```python
from build123d import *

# Parameters (mm, degrees)
FILLET1_R   = 0.1
FILLET2_R   = 0.15
HEX_2_DEPTH = 1.3


with BuildPart() as part:
    # BodySke → Base-Revolve (revolve)
    with BuildSketch(Plane.XY, mode=Mode.PRIVATE) as base_revolve_sk:
        Polygon((0, 0), (0, 2.75), (3, 2.75), (3, 1.5), (18.7195, 1.5), (19, 1.2195), (19, 0), align=None)
    revolve(base_revolve_sk.sketch.rotate(Axis((-31.75, 0, 0), (1, 0, 0)), 90), axis=Axis((-31.75, 0, 0), (1, 0, 0)))  # turned: the seam where the file's is

    # Fillet1
    fillet1_edges = [part.edges().sort_by_distance(p)[0] for p in [
        (3, 0, -1.5),
    ]]
    fillet(fillet1_edges, radius=FILLET1_R)

    # Fillet2
    fillet2_edges = [part.edges().sort_by_distance(p)[0] for p in [
        (0, 0, -2.75),
    ]]
    fillet(fillet2_edges, radius=FILLET2_R)

    # Sketch2 → Hex-PreBroach (revolve, cut)
    with BuildSketch(Plane.XY, mode=Mode.PRIVATE) as hex_prebroach_sk:
        Polygon((0, 1.28), (1.3, 1.28), (2.039008345, 0), (0, 0), align=None)
    revolve(hex_prebroach_sk.sketch.rotate(Axis((0, 0, 0), (1, 0, 0)), 90), axis=Axis((0, 0, 0), (1, 0, 0)), mode=Mode.SUBTRACT)  # turned: the seam where the file's is

    # Sketch3 → Hex 2 (cut)
    with BuildSketch(Plane(origin=(0, 0, 0), x_dir=(0, 0.5, 0.866025404), z_dir=(-1, 0, 0))):
        Polygon((0.739008345, 1.28), (-0.739008345, 1.28), (-1.478016689, 0), (-0.739008345, -1.28), (0.739008345, -1.28), (1.478016689, 0), align=None)
    extrude(amount=-HEX_2_DEPTH, mode=Mode.SUBTRACT)


solid = part.part
```
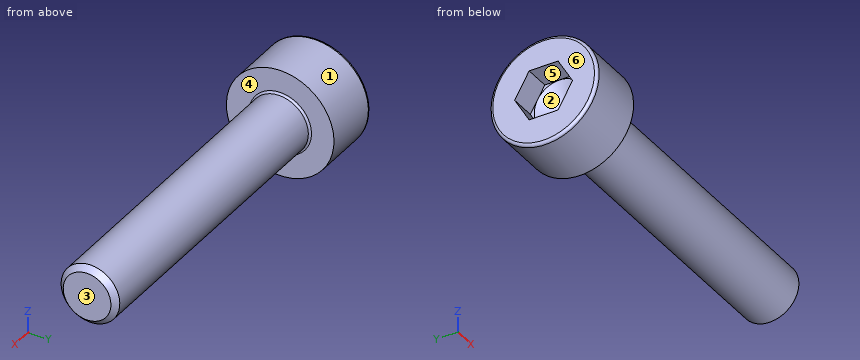
Here's how the part is built. I have some questions about the finished solid (model axes, mm). Face numbers are marked on the shaded views. A direction names the side the tool comes from. Round coordinates to 2 decimals unless told otherwise and drop trailing zeros. Order: outer loops, then holes, each group sorted by start corner. A loop starts at its lowest first (then second) coordinate and runs counter-clockwise, first axis right, second up. Notation, with made-up numbers: (-2.5, 40.5) -> (48.5, 40.5) arc R32 ccw to (48.5, 71.5) -> close; hole circle Ø4 at (44, 83.5). An arc over 180 degrees is marked (long way). Use a Markdown table: item, result. Add a question column.
(1) For the marked faces 4, 5 and 6, which set-ups out of +Z, -Z, +X, -X, +Y, -Y let a thin tool reach every point of the face, with its end or its side?
(2) I need wall thicknesses on line 1 along X through (y, z) = (-0.35, -1.85); line 2 along Z through (x, y) = (1, -1); line 3 along Y through (x, z) = (6, -0.05). Which ranges of each line are inside material? Lowest first, please.
(3) If we mould it in two halves opening along Z, with no side actions, what happens to the marked faces 1, 2 and 3? For each: released by +Z, released by -Z, zero draft, split by the parting line, or undercut.
(4) Suppose I cut it at A-A, the plane x = 13.5. Please give me the cut outline in (y, z), and give its area (3 significant figures).
(5) For pin 1 Ø0.5 at (y, z) = (-0.5, 1) entering from -X; pin 2 Ø3 at (x, y) = (17, 0.5) entering from -Z, each with a flat end and sliding along its axis, tell me the tip position at first contact or that it passes through.
Verdict:
| question | item | result |
|---|---|---|
| 1 | face 4 | +X |
| 1 | face 5 | -X |
| 1 | face 6 | +Z, -Z, -X, +Y, -Y |
| 2 | line 1 | 0 to 3 |
| 2 | line 2 | -2.56 to -0.83, 0.83 to 2.56 |
| 2 | line 3 | -1.5 to 1.5 |
| 3 | face 1 | split by the parting line |
| 3 | face 2 | undercut |
| 3 | face 3 | zero draft |
| 4 | outline | circle Ø3 at (0, 0) |
| 4 | area | 7.07 mm2 |
| 5 | pin 1 | x = 1.3 |
| 5 | pin 2 | z = -1.5 |
